```python
from build123d import *

# Parameters (mm, degrees)
SKETCH1_R           = 30
BOSS_EXTRUDE1_DEPTH = 25
DRAFT1_ANGLE        = -10
SHELL2_T            = -3
SKETCH1_4_R         = 8.5
CUT_EXTRUDE2_DEPTH  = 3


with BuildPart() as part:
    # Sketch1 → Boss-Extrude1 (new body)
    with BuildSketch(Plane(origin=(0, 0, 0), x_dir=(1, 0, 0), z_dir=(0, 1, 0))):
        with Locations(Location((0, 0, 0), (0, 0, 270))):
            Circle(SKETCH1_R)
    extrude(amount=-BOSS_EXTRUDE1_DEPTH)

    # Draft1
    draft1_faces = [part.faces().sort_by_distance(p)[0] for p in [
        (0, -12.5, -30),
    ]]
    draft(draft1_faces, Plane.ZX, DRAFT1_ANGLE)

    # Shell2
    shell2_openings = [part.faces().sort_by_distance(p)[0] for p in [
        (0, -25, 0),
    ]]
    offset(amount=SHELL2_T, openings=shell2_openings, kind=Kind.INTERSECTION)

    # Sketch1<4> → Cut-Extrude2 (cut)
    with BuildSketch(Plane(origin=(0, 0, 0), x_dir=(1, 0, 0), z_dir=(0, 1, 0))):
        with Locations(Location((-13, 0, 0), (0, 0, 270))):
            Circle(SKETCH1_4_R)
        with Locations(Location((13, 0, 0), (0, 0, 270))):
            Circle(SKETCH1_4_R)
    extrude(amount=-CUT_EXTRUDE2_DEPTH, mode=Mode.SUBTRACT)


solid = part.part
```
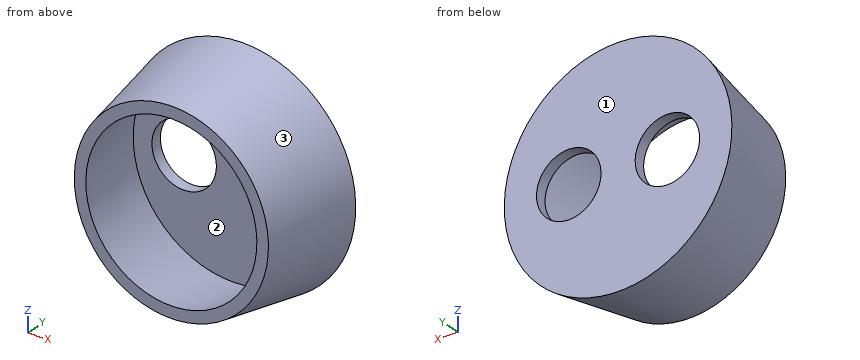
Input: part model. Units: mm. Frame: model coordinates. Face numbers are marked on the shaded views. Give positions to 0.01 mm unless a question says otherwise; leave off trailing zeros. Order: outer loops, then holes, each group sorted by start corner. A loop starts at its lowest first (then second) coordinate and runs counter-clockwise, first axis right, second up. Notation, with made-up numbers: M 8,-9.75 L 61,-9.75 A21 cw 61,5.25 Z; hole C -27,69 d3. An arc over 180 degrees is marked long. Return JSON: item names as keys, results as strings.
Item 1: Cut plane B-B (x = 0). Return loops of the section in (y, z), then the cut area to 3 significant figures.
Solutions:
{"outline": "M -25,-25.59 L 0,-30 L 0,30 L -25,25.59 L -25,22.55 L -3,26.42 L -3,-26.42 L -25,-22.55 Z", "area": "312 mm^2"}
Item 2: Pull-direction query (X, two-part tool) for the marked faces 1, 2 and 3; classes: +X half, -X half, draft (parallel to the pull), parting line (faces both ways), or undercut.
Solutions:
{"face 1": "draft", "face 2": "undercut", "face 3": "parting line"}
Item 3: First-contact query: P1, Ø3, axis at x = 13, y = -15.5, coming from the -Z side; P2, Ø5, axis at x = -17.5, y = -6.5, coming from the +Z side; P3, Ø8, axis at y = -10.5, z = 5, coming from the +X side. Flat tips, straight axial feed; report the tip coordinate or a pass-through.
Solutions:
{"P1": "z = -24.78", "P2": "z = 24.73", "P3": "x = 28.6"}
Item 4: Cut plane C-C (y = -21). Return loops of the section in (x, z).
Solutions:
{"outline": "C 0,0 d52.59; hole C 0,0 d46.5"}
Item 5: Ray query, probe 1 along X at (y, z) = (-2.25, 0); probe 2 along X at (y, z) = (-1.9, 0); probe 3 along Y at (x, z) = (-19.5, 6.5). Return the intervals inside material, ascending.
Solutions:
{"probe 1": "-29.6 to -21.5, -4.5 to 4.5, 21.5 to 29.6", "probe 2": "-29.66 to -21.5, -4.5 to 4.5, 21.5 to 29.66", "probe 3": "-3 to 0"}
Item 6: Cut plane A-A (z = 0). Return loops of the section in (x, y), then the cut area to 3 significant figures.
Solutions:
{"outline": "M -30,0 L -25.59,-25 L -22.55,-25 L -26.42,-3 L -21.5,-3 L -21.5,0 Z; M -4.5,-3 L 4.5,-3 L 4.5,0 L -4.5,0 Z; M 21.5,-3 L 26.42,-3 L 22.55,-25 L 25.59,-25 L 30,0 L 21.5,0 Z", "area": "210 mm^2"}
Item 7: Cut plane D-D (y = -10.75). Return loops of the section in (x, z).
Solutions:
{"outline": "C 0,0 d56.21; hole C 0,0 d50.12"}
